from build123d import *

# Parameters (mm, degrees)
F2_W     = 7
F2_H     = 7
F3_DEPTH = 42.001
F5_D     = 10
F6_SIZE  = 1
F7_SIZE  = 0.5
F8_SIZE  = 1
F9_R     = 1
F10_R    = 2
F11_R    = 0.5


with BuildPart() as f1:
    # F0 (on Right) → F1 (revolve)
    with BuildSketch(Plane.YZ):
        Polygon((0, 12), (0, 20), (-2, 20), (-2, 56), (-18, 56), (-18, 22.5), (-42, 22.5), (-42, 12), align=None)
    revolve(axis=Axis((0, -17.673691, 0), (0, 1, 0)))

    # F2 (on face) → F3 (cut, through all)
    with BuildSketch(Plane.XZ.offset(42)):
        with Locations((0, 11.5)):
            Rectangle(F2_W, F2_H)
    extrude(amount=-F3_DEPTH, mode=Mode.SUBTRACT)

    # F5 (through all)
    with Locations(Plane.XZ.offset(18)):
        with Locations((26.516504, 26.516504), (26.516504, -26.516504), (-26.516504, 26.516504), (-26.516504, -26.516504)):
            Hole(F5_D / 2)

    # F6
    f6_edges = [f1.edges().sort_by_distance(p)[0] for p in [
        (3.5, -42, 13.23912),
        (3.5, 0, 13.23912),
        (-3.5, 0, 13.23912),
        (0, 0, 15),
        (0, 0, -12),
        (0, -42, -12),
        (-3.5, -42, 13.23912),
        (0, -42, 15),
    ]]
    chamfer(f6_edges, length=F6_SIZE)

    # F7
    f7_edges = [f1.edges().sort_by_distance(p)[0] for p in [
        (0, 0, -20),
    ]]
    chamfer(f7_edges, length=F7_SIZE)

    # F8
    f8_edges = [f1.edges().sort_by_distance(p)[0] for p in [
        (0, -2, -56),
    ]]
    chamfer(f8_edges, length=F8_SIZE)

    # F9
    f9_edges = [f1.edges().sort_by_distance(p)[0] for p in [
        (0, -18, -56),
    ]]
    fillet(f9_edges, radius=F9_R)

    # F10
    f10_edges = [f1.edges().sort_by_distance(p)[0] for p in [
        (0, -18, -22.5),
        (0, -42, -22.5),
    ]]
    fillet(f10_edges, radius=F10_R)

    # F11
    f11_edges = [f1.edges().sort_by_distance(p)[0] for p in [
        (0, -2, -20),
    ]]
    fillet(f11_edges, radius=F11_R)


solid = f1.part
Read the model definition and answer for the solid it produces. Units are mm, in the model's axes. A direction names the side the tool comes from. Round coordinates to 2 decimals unless told otherwise and drop trailing zeros. Write each loop counter-clockwise with the first axis right and the second up, starting at its lowest first coordinate (ties: lowest second). Pieces come first, ordered by that corner, then holes.
1. Given pin 1 Ø1 at (x, y) = (21, -17.5) entering from -Z; pin 2 Ø13 at (x, z) = (26.52, 26.52) entering from +Y; pin 3 Ø10 at (y, z) = (-33, -21.5) entering from +X, each flat-ended and moving along its own axis, determine where each tip first touches the part or whether it passes through.
2. Straight lines are drawn through the part: L1, parallel to X at y = -10, z = 0; L2, parallel to Y at x = 38, z = 3; L3, parallel to Z at x = 25.5, y = -10.5. For each, find the intervals that lie inside material, in ascending order.
3. The part is cut by section C-C, the plane y = -34. Determine the outline of the cut face in (x, z), then the cut area to 3 significant figures.
4. Which of the six approach directions +Z, -Z, +X, -X, +Y, -Y give full straight-line access (tool end or side, diameter ignored) to faces 4 (the face through (-4, 0, -13)), 5 (the face through (-19.524, -1.007, -4.336)), 6 (the face through (-24, -18, 11)), 7 (the face through (3.5, -21, 13))?
5. The part is cut by section D-D, the plane y = -11.5. Determine the outline of the cut face in (x, z).
6. Determine the mould class of faces 1 (the face through (-13.4, -42, -0.3)), 2 (the face through (0, -21, -12)), 3 (the face through (-19.961, -30.14, 10.382)) for opening direction Z: pulls with the +Z half, pulls with the -Z half, needs draft (parallel to the pull), parting line crosses it, or undercut.
Values:
1. pin 1: stops at z = -52.05
1. pin 2: stops at y = -2
1. pin 3: stops at x = 15.3
2. L1: x = -56 to -12, 12 to 56
2. L2: y = -18 to -2
2. L3: z = -49.86 to -31.41, -21.62 to 21.62, 31.41 to 49.86
3. outline: circle Ø45 at (0, 0); hole (-3.5, 11.48) arc R12 ccw (long way) to (3.5, 11.48) - (3.5, 15) - (-3.5, 15) - close
3. area: 1,120 mm2
4. face 4: +Z, -Z, +X, -X, +Y
4. face 5: +Y
4. face 6: -Y
4. face 7: +Y, -Y
5. outline: circle Ø112 at (0, 0); hole circle Ø10 at (-26.52, -26.52); hole circle Ø10 at (-26.52, 26.52); hole (-3.5, 11.48) arc R12 ccw (long way) to (3.5, 11.48) - (3.5, 15) - (-3.5, 15) - close; hole circle Ø10 at (26.52, -26.52); hole circle Ø10 at (26.52, 26.52)
6. face 1: needs draft
6. face 2: undercut
6. face 3: parting line crosses it
